Read the model definition and answer for the solid it produces. Units are mm, in the model's axes. A direction names the side the tool comes from. Coordinates: 2 decimals unless noted, no trailing zeros. Order: outer loops, then holes, each group sorted by start corner. A loop starts at its lowest first (then second) coordinate and runs counter-clockwise, first axis right, second up. Notation, with made-up numbers: (26.25, 43.25) - (31.25, 43.25) arc R13 cw to (31.25, 54.25) - close; hole circle Ø10 at (-32, -30.5). An arc over 180 degrees is marked (long way). Use one line per item in the form item = value. Start each with the question number.
from build123d import *

# Parameters (mm, degrees)
BOSS_EXTRUDE1_DEPTH = 72.5


with BuildPart() as part:
    # Sketch1 → Boss-Extrude1 (new, symmetric)
    with BuildSketch(Plane.XY):
        Polygon((-10, 3), (-10, 10), (-3, 10), (-3, 8.27), (-5.78, 8.27), (-5.78, 6.75), (-3, 4.542263603), (3, 4.542263603), (5.78, 6.75), (5.78, 8.27), (3, 8.27), (3, 10), (10, 10), (17, 10), (17, 8.27), (14.22, 8.27), (14.22, 6.75), (17, 4.542263603), (23, 4.542263603), (25.78, 6.75), (25.78, 8.27), (23, 8.27), (23, 10), (30, 10), (37, 10), (37, 8.27), (34.22, 8.27), (34.22, 6.75), (37, 4.542263603), (43, 4.542263603), (45.78, 6.75), (45.78, 8.27), (43, 8.27), (43, 10), (50, 10), (57, 10), (57, 8.27), (54.22, 8.27), (54.22, 6.75), (57, 4.542263603), (63, 4.542263603), (65.78, 6.75), (65.78, 8.27), (63, 8.27), (63, 10), (70, 10), (70, 3), (68.27, 3), (68.27, 5.78), (66.75, 5.78), (64.542263603, 3), (64.542263603, -3), (66.75, -5.78), (68.27, -5.78), (68.27, -3), (70, -3), (70, -10), (63, -10), (63, -8.27), (65.78, -8.27), (65.78, -6.75), (63, -4.542263603), (57, -4.542263603), (54.22, -6.75), (54.22, -8.27), (57, -8.27), (57, -10), (50, -10), (43, -10), (43, -8.27), (45.78, -8.27), (45.78, -6.75), (43, -4.542263603), (37, -4.542263603), (34.22, -6.75), (34.22, -8.27), (37, -8.27), (37, -10), (30, -10), (23, -10), (23, -8.27), (25.78, -8.27), (25.78, -6.75), (23, -4.542263603), (17, -4.542263603), (14.22, -6.75), (14.22, -8.27), (17, -8.27), (17, -10), (10, -10), (3, -10), (3, -8.27), (5.78, -8.27), (5.78, -6.75), (3, -4.542263603), (-3, -4.542263603), (-5.78, -6.75), (-5.78, -8.27), (-3, -8.27), (-3, -10), (-10, -10), (-10, -3), (-8.27, -3), (-8.27, -5.78), (-6.75, -5.78), (-4.542263603, -3), (-4.542263603, 3), (-6.75, 5.78), (-8.27, 5.78), (-8.27, 3), align=None)
    extrude(amount=BOSS_EXTRUDE1_DEPTH, both=True)


solid = part.part
Q1. For a pull along X with two mould halves and no side action, classify faces 1 (the flat face through (10, -10, 1)), 2 (the flat face through (24.41, -5.66, 1.02)), 3 (the flat face through (-10, -7, 1)) as +X half, -X half, draft (parallel to the pull), parting line (faces both ways), or undercut.
Q2. A cutting plane is placed at B-B (x = -1). Give the vertices of the cut face in (y, z), then the cut area to 3 significant figures.
Q3. Which of the six approach directions +Z, -Z, +X, -X, +Y, -Y give full straight-line access (tool end or side, diameter ignored) to faces 4 (the flat face through (60, -4.542, 1)), 5 (the flat face through (24, 8.27, 1)), 6 (the flat face through (70, -6, 1))?
Q4. Given P1, Ø6.5, axis at x = 1, z = -18.5, coming from the +Y side; P2, Ø3, axis at y = -1, z = 35.5, coming from the +X side; P3, Ø1, axis at x = 38, z = 47, coming from the -Y side; P4, Ø2, axis at x = 61, z = 7.5, coming from the +Y side, each flat-ended and moving along its own axis, determine where each tip first touches the part or whether it passes through.
Q5. A cutting plane is placed at A-A (y = 0.25). Give the vertices of the cut face in (x, z), then the cut area to 3 significant figures.
Q6. Consider probe 1 along X at (y, z) = (7.25, 2); probe 2 along Y at (x, z) = (63.5, -7); probe 3 along Y at (x, z) = (-5, 30). Determine where each line is inside the solid, lowest interval first.
Result sheet:
q1.face_1 = draft
q1.face_2 = undercut
q1.face_3 = -X half
q2.outline = (-4.54, -72.5) - (4.54, -72.5) - (4.54, 72.5) - (-4.54, 72.5) - close
q2.area = 1,320 mm^2
q3.face_4 = +Z, -Z, -Y
q3.face_5 = +Z, -Z
q3.face_6 = +Z, -Z, +X, +Y, -Y
q4.P1 = 10
q4.P2 = 64.54
q4.P3 = -4.54
q4.P4 = 4.54
q5.outline = (-4.54, -72.5) - (64.54, -72.5) - (64.54, 72.5) - (-4.54, 72.5) - close
q5.area = 10,000 mm^2
q6.probe_1 = -10 to -5.78, 5.78 to 14.22, 25.78 to 34.22, 45.78 to 54.22, 65.78 to 70
q6.probe_2 = -10 to -8.27, -4.94 to 4.94, 8.27 to 10
q6.probe_3 = -10 to -8.27, -6.13 to -3.58, 3.58 to 6.13, 8.27 to 10
